from build123d import *

# Parameters (mm, degrees)
F3_SIZE  = 5.08
F5_DEPTH = 25.4


# Not quite as in the source:
# - a fillet or chamfer that OpenCascade refuses, or shapes differently, is made with other operations: its cross-section is extruded or revolved along the edge and cut away or added


with BuildPart() as f1:
    # F0 (on Top) → F1 (revolve)
    with BuildSketch(Plane.XY):
        Polygon((-19.9900865555, -40.7797805965), (-19.9900865555, 45.5773994327), (-51.6543835402, 45.5773994327), (-43.658349663, 28.9456453174), (-27.9861204326, 28.9456453174), (-23.8281842321, -19.3504039198), (-43.0186651647, -30.8646950871), (-43.0186651647, -43.3385074139), align=None)
    revolve(axis=Axis((0, -1.2793652713, 0), (0, -1, 0)))

    # F2: fillet of radius 15.0328655844 on 1 edges, made by hand

    # F2_s1 → F2_t2 (revolve, cut)
    with BuildSketch(Plane.XY):
        with BuildLine():
            ThreePointArc((-28.7107544335, 45.5773994327), (-39.8916069066, 40.5931947369), (-43.658349663, 28.9456453174))
            Line((-43.658349663, 28.9456453174), (-51.6543835402, 45.5773994327))
            Line((-51.6543835402, 45.5773994327), (-28.7107544335, 45.5773994327))
        make_face()
    revolve(axis=Axis((0, 45.5773994327, 0), (0, -1, 0)), mode=Mode.SUBTRACT)

    # F3
    f3_edges = [f1.edges().sort_by_distance(p)[0] for p in [
        (43.018665, -43.338507, 0),
    ]]
    chamfer(f3_edges, length=F3_SIZE)

    # F4 (on face) → F5 (join)
    with BuildSketch(Plane(origin=(0, 45.5773994327, 0), x_dir=(-1, 0, 0), z_dir=(0, 1, 0))):
        with BuildLine():
            ThreePointArc((1.7598816693, -28.6567659838), (12.6790964927, -25.7594241448), (21.635263345, -18.8738655324))
            ThreePointArc((21.635263345, -18.8738655324), (18.1448647045, -15.8726036273), (13.7469387774, -14.5129333612))
            ThreePointArc((13.7469387774, -14.5129333612), (8.8279197581, -17.9351998383), (3.1156176835, -19.7457966906))
            ThreePointArc((3.1156176835, -19.7457966906), (1.5105456445, -24.0602143155), (1.7598816693, -28.6567659838))
        make_face()
    extrude(amount=F5_DEPTH)


solid = f1.part
Read the model definition and answer for the solid it produces. Units are mm, in the model's axes. A direction names the side the tool comes from. Coordinates: 2 decimals unless noted, no trailing zeros. Order: outer loops, then holes, each group sorted by start corner. A loop starts at its lowest first (then second) coordinate and runs counter-clockwise, first axis right, second up. Notation, with made-up numbers: (76, 81) - (100, 81) arc R16 ccw to (100, 104) - close; hole circle Ø6 at (-32.5, -13.5). An arc over 180 degrees is marked (long way). Use one line per item in the form item = value.
(1) Given pin 1 Ø3 at (y, z) = (-14.5, -10.5) entering from -X; pin 2 Ø2 at (x, z) = (29, 12.5) entering from +Y; pin 3 Ø4 at (x, y) = (31.5, 43) entering from +Z, each flat-ended and moving along its own axis, determine where each tip first touches the part or whether it passes through.
Computed values:
pin_1 = -22.53
pin_2 = 45.46
pin_3 = 24.73
(2) For a pull along Y with two mould halves and no side action, classify faces 1 (the face through (-19.9, -40.877, -6.267)), 2 (the face through (-23.12, -20.07, 9.59)), 3 (the face through (13, 45.577, 17)), 4 (the face through (-1.52, 58.1, -24)) as pulls with the +Y half, pulls with the -Y half, needs draft (parallel to the pull), parting line crosses it, or undercut.
Computed values:
face_1 = pulls with the -Y half
face_2 = undercut
face_3 = pulls with the +Y half
face_4 = needs draft
(3) Section A-A, the plane y = -26.5 is taken. Give the vertices of the cut face in (x, z).
Computed values:
outline = circle Ø71.49 at (0, 0); hole circle Ø39.98 at (0, 0)
(4) Straight lines are drawn through the part: L1, parallel to X at y = 9, z = 0; L2, parallel to Z at x = 0, y = 1; L3, parallel to Z at x = 0, y = -22.5. For each, find the intervals that lie inside material, in ascending order.
Computed values:
L1 = -26.27 to -19.99, 19.99 to 26.27
L2 = -25.58 to -19.99, 19.99 to 25.58
L3 = -29.08 to -19.99, 19.99 to 29.08
(5) Section B-B, the plane y = 13.5 is taken. Give the vertices of the cut face in (x, z), then the cut area to 3 significant figures.
Computed values:
outline = circle Ø53.31 at (0, 0); hole circle Ø39.98 at (0, 0)
area = 977 mm²
(6) Which of the six approach directions +Z, -Z, +X, -X, +Y, -Y give full straight-line access (tool end or side, diameter ignored) to faces 5 (the face through (-12.536, 58.1, -25.829)), 6 (the face through (9.3, -34.6, 42)), 7 (the face through (-11, 70.977, -21)), 8 (the face through (-18.202, 58.1, -15.904)), 9 (the face through (-28.5, 28.946, -0.6))?
Computed values:
face_5 = -Z, -X, +Y
face_6 = -Y
face_7 = +Z, -Z, +X, -X, +Y
face_8 = +Z, -X, +Y
face_9 = none
